Source: CAD feature listing. Evaluate the final solid. Frame: model axes, mm. Face numbers are marked on the shaded views. A direction names the side the tool comes from. Coordinates: 2 decimals unless noted, no trailing zeros. Write each loop counter-clockwise with the first axis right and the second up, starting at its lowest first coordinate (ties: lowest second). Pieces come first, ordered by that corner, then holes. Notation, with made-up numbers: (64, 46) - (78, 46) arc R13 ccw to (78, 62) - close; hole circle Ø2 at (72, 40). An arc over 180 degrees is marked (long way). One line per question, with ' | ' between items.
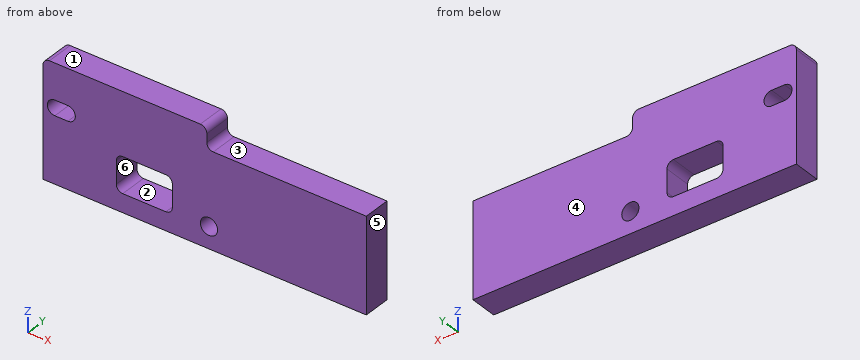
from build123d import *

# Parameters (mm, degrees)
SKETCH1_R           = 2
SKETCH1_R_2         = 3
SKETCH1_W           = 13
SKETCH1_H           = 8.25
BOSS_EXTRUDE1_DEPTH = 6.35
FILLET1_R           = 1.5
SKETCH2_W           = 82.327825706
SKETCH2_H           = 14.458254131
CUT_EXTRUDE1_DEPTH  = 51
SKETCH3_W           = 51.5
SKETCH3_H           = 6.35
BOSS_EXTRUDE2_DEPTH = 25
SKETCH4_W           = 84.929028447
SKETCH4_H           = 25.885902506
CUT_EXTRUDE2_DEPTH  = 90
SKETCH5_W           = 0.1
SKETCH5_H           = 6.35
CUT_EXTRUDE3_DEPTH  = 90
SKETCH6_W           = 81.24526446
SKETCH6_H           = 21.013173112
CUT_EXTRUDE4_DEPTH  = 71


with BuildPart() as part:
    # Sketch1 → Boss-Extrude1 (new body)
    with BuildSketch(Plane(origin=(0, 0, 0), x_dir=(1, 0, 0), z_dir=(0, 1, 0))):
        Polygon((38, 0), (38, 5), (58, 5), (58, 0), (96, 0), (96, 48.5), (89, 58.5), (89, 67.5), (62, 67.5), (62, 56.5), (34, 56.5), (34, 67.5), (7, 67.5), (7, 58.5), (0, 48.5), (0, 0), align=None)
        with Locations(Location((38.5, 40, 0), (0, 0, 270))):
            Circle(SKETCH1_R, mode=Mode.SUBTRACT)
        with Locations(Location((38.5, 22, 0), (0, 0, 270))):
            Circle(SKETCH1_R, mode=Mode.SUBTRACT)
        with Locations(Location((57.5, 22, 0), (0, 0, 90))):
            Circle(SKETCH1_R, mode=Mode.SUBTRACT)
        with Locations(Location((57.5, 40, 0), (0, 0, 90))):
            Circle(SKETCH1_R, mode=Mode.SUBTRACT)
        with Locations(Location((12.5, 61.75, 0), (0, 0, 270))):
            Circle(SKETCH1_R_2, mode=Mode.SUBTRACT)
        with Locations(Location((28, 61.75, 0), (0, 0, 270))):
            Circle(SKETCH1_R_2, mode=Mode.SUBTRACT)
        with Locations(Location((68, 61.75, 0), (0, 0, 90))):
            Circle(SKETCH1_R_2, mode=Mode.SUBTRACT)
        with Locations(Location((83.5, 61.75, 0), (0, 0, 90))):
            Circle(SKETCH1_R_2, mode=Mode.SUBTRACT)
        with Locations((72.5, 18.625)):
            Rectangle(SKETCH1_W, SKETCH1_H, mode=Mode.SUBTRACT)
        with Locations((23.5, 34.875)):
            Rectangle(SKETCH1_W, SKETCH1_H, mode=Mode.SUBTRACT)
        with Locations((23.5, 18.625)):
            Rectangle(SKETCH1_W, SKETCH1_H, mode=Mode.SUBTRACT)
        with Locations((72.5, 34.875)):
            Rectangle(SKETCH1_W, SKETCH1_H, mode=Mode.SUBTRACT)
        with BuildLine():
            Line((2.75, 11.75), (5.75, 11.75))
            ThreePointArc((5.75, 11.75), (7.5, 10), (5.75, 8.25))
            Line((5.75, 8.25), (2.75, 8.25))
            ThreePointArc((2.75, 8.25), (1, 10), (2.75, 11.75))
        make_face(mode=Mode.SUBTRACT)
        with BuildLine():
            Line((93.25, 8.25), (90.25, 8.25))
            ThreePointArc((90.25, 8.25), (88.5, 10), (90.25, 11.75))
            Line((90.25, 11.75), (93.25, 11.75))
            ThreePointArc((93.25, 11.75), (95, 10), (93.25, 8.25))
        make_face(mode=Mode.SUBTRACT)
        with BuildLine():
            Line((93.25, 45.5), (90.25, 45.5))
            ThreePointArc((90.25, 45.5), (88.5, 47.25), (90.25, 49))
            Line((90.25, 49), (93.25, 49))
            ThreePointArc((93.25, 49), (95, 47.25), (93.25, 45.5))
        make_face(mode=Mode.SUBTRACT)
        with BuildLine():
            Line((2.75, 49), (5.75, 49))
            ThreePointArc((5.75, 49), (7.5, 47.25), (5.75, 45.5))
            Line((5.75, 45.5), (2.75, 45.5))
            ThreePointArc((2.75, 45.5), (1, 47.25), (2.75, 49))
        make_face(mode=Mode.SUBTRACT)
    extrude(amount=BOSS_EXTRUDE1_DEPTH)

    # Fillet1
    fillet1_edges = [part.edges().sort_by_distance(p)[0] for p in [
        (0, 3.175, -48.5),
        (7, 3.175, -58.5),
        (7, 3.175, -67.5),
        (34, 3.175, -67.5),
        (34, 3.175, -56.5),
        (62, 3.175, -56.5),
        (62, 3.175, -67.5),
        (89, 3.175, -67.5),
        (89, 3.175, -58.5),
        (96, 3.175, -48.5),
        (96, 3.175, 0),
        (58, 3.175, 0),
        (58, 3.175, -5),
        (38, 3.175, -5),
        (38, 3.175, 0),
        (0, 3.175, 0),
        (17, 3.175, -39),
        (17, 3.175, -30.75),
        (30, 3.175, -30.75),
        (30, 3.175, -39),
        (17, 3.175, -22.75),
        (17, 3.175, -14.5),
        (30, 3.175, -14.5),
        (30, 3.175, -22.75),
        (79, 3.175, -14.5),
        (79, 3.175, -22.75),
        (66, 3.175, -22.75),
        (66, 3.175, -14.5),
        (79, 3.175, -30.75),
        (79, 3.175, -39),
        (66, 3.175, -39),
        (66, 3.175, -30.75),
    ]]
    fillet(fillet1_edges, radius=FILLET1_R)

    # Sketch2 → Cut-Extrude1 (cut)
    with BuildSketch(Plane(origin=(48, 0, 0), x_dir=(0, 0, -1), z_dir=(1, 0, 0))):
        with Locations((33.293792952, 1.315835649)):
            Rectangle(SKETCH2_W, SKETCH2_H)
    extrude(amount=CUT_EXTRUDE1_DEPTH, mode=Mode.SUBTRACT)

    # Sketch3 → Boss-Extrude2 (add)
    with BuildSketch(Plane(origin=(48, 0, 0), x_dir=(0, 0, -1), z_dir=(1, 0, 0))):
        with Locations((30.75, 3.175)):
            Rectangle(SKETCH3_W, SKETCH3_H)
    extrude(amount=BOSS_EXTRUDE2_DEPTH)

    # Mirror1: part across plane


with BuildPart() as part_1:
    add(part.part)
    add(part.part.mirror(Plane(origin=(73, 0, 0), x_dir=(0, 0, 1), z_dir=(1, 0, 0))))

    # Sketch4 → Cut-Extrude2 (cut)
    with BuildSketch(Plane(origin=(75, 0, 0), x_dir=(0, 0, -1), z_dir=(1, 0, 0))):
        with Locations((34.029781947, 1.13903014)):
            Rectangle(SKETCH4_W, SKETCH4_H)
    extrude(amount=CUT_EXTRUDE2_DEPTH, mode=Mode.SUBTRACT)

    # Sketch5 → Cut-Extrude3 (cut)
    with BuildSketch(Plane(origin=(75, 0, 0), x_dir=(0, 0, -1), z_dir=(1, 0, 0))):
        with Locations((27.05, 3.175)):
            Rectangle(SKETCH5_W, SKETCH5_H)
    extrude(amount=-CUT_EXTRUDE3_DEPTH, mode=Mode.SUBTRACT)


with BuildPart() as cut_extrude3_piece_1:
    # of the separate pieces the step leaves, piece 1, a body of its own (cut_extrude3_pieces)
    add(part_1.part.solids().sort_by_distance((0, 0, -48.027166654))[0])

    # Sketch6 → Cut-Extrude4 (cut)
    with BuildSketch(Plane(origin=(0, 0, -27), x_dir=(-1, 0, 0), z_dir=(0, 0, -1))):
        with Locations((-35.926138856, 1.728749219)):
            Rectangle(SKETCH6_W, SKETCH6_H)
    extrude(amount=CUT_EXTRUDE4_DEPTH, mode=Mode.SUBTRACT)


with BuildPart() as cut_extrude3_piece_2:
    # of the separate pieces the step leaves, piece 2, a body of its own (cut_extrude3_pieces)
    add(part_1.part.solids().sort_by_distance((38, 0, -1.5))[0])


solid = cut_extrude3_piece_2.part
Item 1: Cut plane A-A on y = 1.5. Return loops of the section in (x, z).
Check sheet entries:
outline: (0, -27) - (75, -27) - (75, -5) - (39.5, -5) arc R1.5 cw to (38, -3.5) - (38, -1.5) arc R1.5 ccw to (36.5, 0) - (1.5, 0) arc R1.5 ccw to (0, -1.5) - close; hole (2.75, -11.75) - (5.75, -11.75) arc R1.75 ccw to (5.75, -8.25) - (2.75, -8.25) arc R1.75 ccw to start; hole (17, -21.25) arc R1.5 ccw to (18.5, -22.75) - (28.5, -22.75) arc R1.5 ccw to (30, -21.25) - (30, -16) arc R1.5 ccw to (28.5, -14.5) - (18.5, -14.5) arc R1.5 ccw to (17, -16) - close; hole circle Ø4 at (38.5, -22)
Item 2: Access query for the marked faces 1, 2 and 3. Directions: +Z, -Z, +X, -X, +Y, -Y. A direction counts if a zero-diameter tool reaches every point of the face in a straight line with its end or side. Return the directions, or none.
Check sheet entries:
face 1: +Z, +X, -X, +Y, -Y | face 2: +Y, -Y | face 3: +Z, +X, +Y, -Y
Item 3: Cut plane D-D on z = -22. Return loops of the section in (x, y).
Check sheet entries:
outline: (0, 0) - (17.2, 0) - (17.2, 6.35) - (0, 6.35) - close; (29.8, 0) - (36.5, 0) - (36.5, 6.35) - (29.8, 6.35) - close; (40.5, 0) - (75, 0) - (75, 6.35) - (40.5, 6.35) - close
Item 4: Pin query (flat end, axial travel): pin 1 Ø2 at (y, z) = (2, -2.5) entering from +X. Return the tip coordinate at first contact, or that it passes through.
Check sheet entries:
pin 1: x = 38
Item 5: Cut plane C-C on z = -9.5. Return loops of the section in (x, y).
Check sheet entries:
outline: (0, 0) - (1.07, 0) - (1.07, 6.35) - (0, 6.35) - close; (7.43, 0) - (75, 0) - (75, 6.35) - (7.43, 6.35) - close
Item 6: Ray query, line 1 along X through (y, z) = (6, -18.75); line 2 along X through (y, z) = (3, -22); line 3 along Z through (x, y) = (46, 5.5). Return the intervals inside material, ascending. Write a range as [from, to].
Check sheet entries:
line 1: [0, 17], [30, 75] | line 2: [0, 17.2], [29.8, 36.5], [40.5, 75] | line 3: [-27, -5]
Item 7: Mould query, pull axis X, two halves, no side actions, for the marked faces 4, 5 and 6. Classes: pulls with the +X half, pulls with the -X half, needs draft (parallel to the pull), parting line crosses it, or undercut.
Check sheet entries:
face 4: needs draft | face 5: pulls with the +X half | face 6: undercut
Item 8: Cut plane B-B on x = 21. Return loops of the section in (y, z), and give its area (3 significant figures).
Check sheet entries:
outline: (0, -27) - (6.35, -27) - (6.35, -22.75) - (0, -22.75) - close; (0, -14.5) - (6.35, -14.5) - (6.35, 0) - (0, 0) - close | area: 119 mm²
